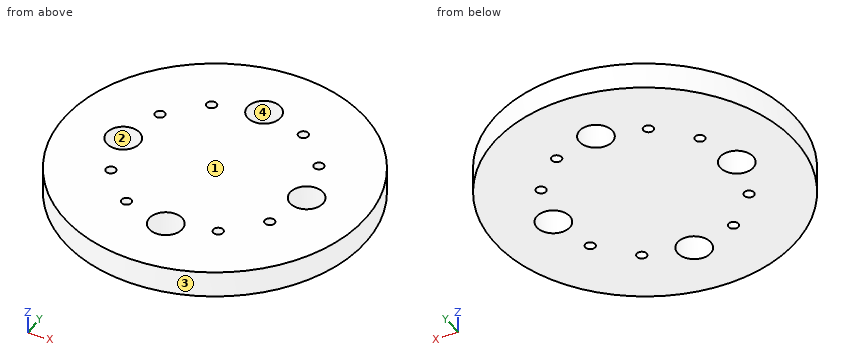
```python
from build123d import *

# Parameters (mm, degrees)
SKETCH_R              = 45.533695
PAD_DEPTH             = 8
SKETCH001_R           = 5
POCKET_DEPTH          = 266.074935
POLARPATTERN_COUNT    = 4
SKETCH002_R           = 1.5
POCKET001_DEPTH       = 266.074935
POLARPATTERN001_COUNT = 12


with BuildPart() as part:
    # Sketch → Pad (new body)
    with BuildSketch(Plane.XY):
        Circle(SKETCH_R)
    extrude(amount=PAD_DEPTH)

    # Sketch001 (on Face3 of Pad) → Pocket (cut, through all)
    with BuildSketch(Plane.XY.offset(8)):
        with Locations((0, 27.533695)):
            Circle(SKETCH001_R)
    pocket = extrude(amount=-POCKET_DEPTH, mode=Mode.SUBTRACT)

    # PolarPattern: Pocket ×4 about axis
    polarpattern_axis = Axis((0, 0, 8), (0, 0, 1))
    for i in range(1, POLARPATTERN_COUNT):
        add(pocket.rotate(polarpattern_axis, i * 360 / POLARPATTERN_COUNT), mode=Mode.SUBTRACT)

    # Sketch002 (on Face3 of Pad) → Pocket001 (cut, through all)
    with BuildSketch(Plane.XY.offset(8)):
        with Locations((-13.766847, 23.844879)):
            Circle(SKETCH002_R)
    pocket001 = extrude(amount=-POCKET001_DEPTH, mode=Mode.SUBTRACT)

    # PolarPattern001: Pocket001 ×12 about axis
    polarpattern001_axis = Axis((0, 0, 8), (0, 0, 1))
    for i in range(1, POLARPATTERN001_COUNT):
        add(pocket001.rotate(polarpattern001_axis, i * 360 / POLARPATTERN001_COUNT), mode=Mode.SUBTRACT)


solid = part.part
```
Verification items for the finished model (mm, model axes). Face numbers are marked on the shaded views. Round coordinates to 2 decimals unless told otherwise and drop trailing zeros. Write each loop counter-clockwise with the first axis right and the second up, starting at its lowest first coordinate (ties: lowest second). Pieces come first, ordered by that corner, then holes. Notation, with made-up numbers: (18.25, -3.75) -> (52.25, -3.75) arc R22 ccw to (52.25, 28.25) -> close; hole circle Ø1 at (-23.5, -23). An arc over 180 degrees is marked (long way). Write each question's results on one line, items separated by ' | '. Start each with the question number.
1. Cross-section at A-A (x = 0). Enter the section's corners in (y, z).
2. Material ranges on probe 1 along Y at (x, z) = (0, 1.5); probe 2 along Y at (x, z) = (15, 2); probe 3 along X at (y, z) = (-24, 1.75), recorded low to high. Write a range as from..to.
3. Draft check along X on the marked faces 1, 2, 3 and 4. Enter one of: +X half, -X half, draft (parallel to the pull), parting line (faces both ways), or undercut.
4. Cross-section at C-C (z = 2.75). Count the separate pieces of the cut face and the enclosed holes in it, then the cut area to 3 significant figures.
5. Depth check by flat-ended pin: P1, Ø6, axis at x = 0, y = 27.53, coming from the +Z side; P2, Ø2, axis at x = 21, z = 5, coming from the -Y side; P3, Ø4, axis at y = -9.5, z = 3.5, coming from the -X side; P4, Ø4, axis at y = -5.5, z = 2.5, coming from the +X side. Enter the tip coordinate at first touch or a pass-through.
6. Cross-section at D-D (y = 29). Enter the section's corners in (x, z), then the cut area to 3 significant figures.
Solutions:
1) outline: (-45.53, 0) -> (-32.53, 0) -> (-32.53, 8) -> (-45.53, 8) -> close; (-22.53, 0) -> (22.53, 0) -> (22.53, 8) -> (-22.53, 8) -> close; (32.53, 0) -> (45.53, 0) -> (45.53, 8) -> (32.53, 8) -> close
2) probe 1: y = -45.53..-32.53, -22.53..22.53, 32.53..45.53 | probe 2: y = -42.99..-24.7, -22.99..22.99, 24.7..42.99 | probe 3: x = -38.7..-15.26, -12.27..-3.54, 3.54..12.27, 15.26..38.7
3) face 1: draft | face 2: undercut | face 3: parting line | face 4: undercut
4) separate pieces: 1 | enclosed holes: 12 | area: 6,140 mm2
5) P1: passes through | P2: stops at y = -40.91 | P3: stops at x = -44.91 | P4: stops at x = 45.4
6) outline: (-35.1, 0) -> (-4.78, 0) -> (-4.78, 8) -> (-35.1, 8) -> close; (4.78, 0) -> (35.1, 0) -> (35.1, 8) -> (4.78, 8) -> close | area: 485 mm2
